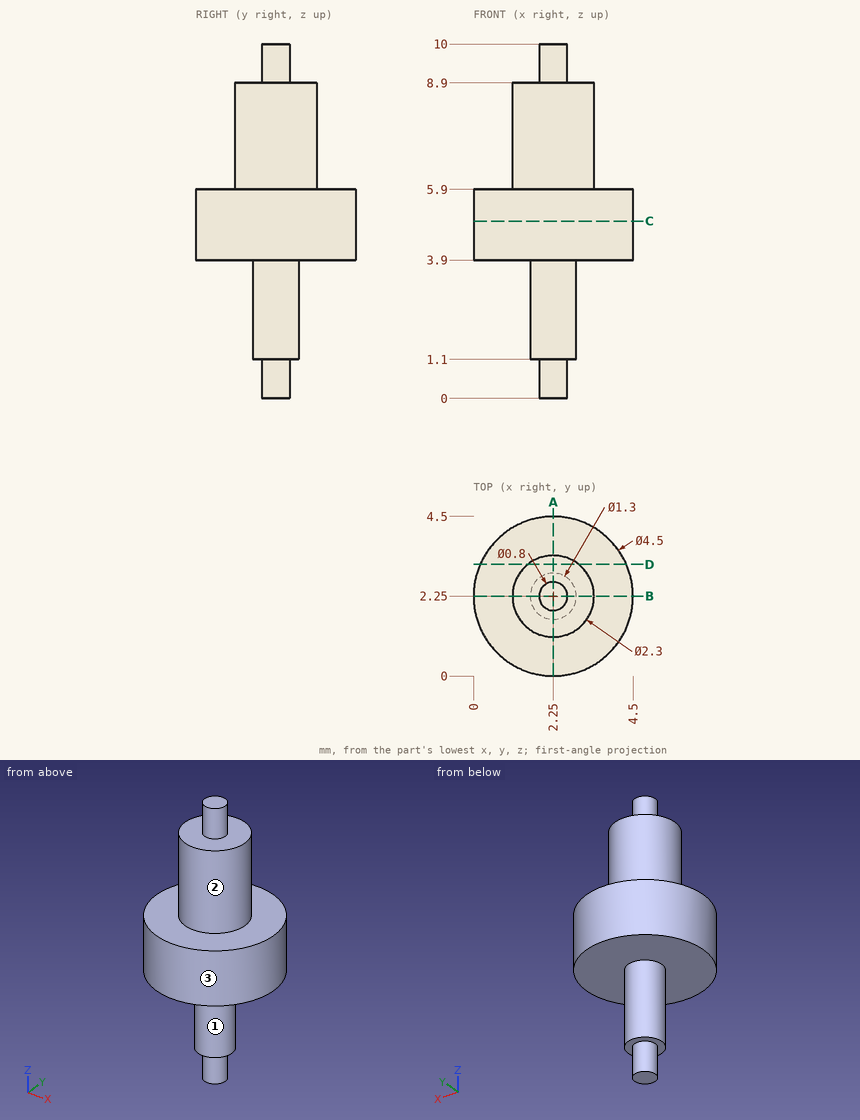
Source: three-view drawing plus pictorial views. Frame: mm from the lowest corner of the part. A direction names the side the tool comes from. Round coordinates to 2 decimals unless told otherwise and drop trailing zeros. Write each loop counter-clockwise with the first axis right and the second up, starting at its lowest first coordinate (ties: lowest second). Pieces come first, ordered by that corner, then holes. Notation, with made-up numbers: M 1.25,56 L 10.25,56 A35 cw 10.25,90 Z; hole C 59.5,7.5 d6. An arc over 180 degrees is marked long. One line per item, written item: value. Start each with the question number.
Item 1: Set-up query: the marked faces 1, 2 and 3. Return all of +Z, -Z, +X, -X, +Y, -Y with unobstructed straight access to the full face (end or side cutting, diameter ignored); none if empty.
Item 2: Section query D-D (y = 3.15). Return the cut outline in (x, z), plus the area to 3 significant figures.
Item 3: Section query A-A (x = 2.25). Return the cut outline in (y, z).
Item 4: Ray query, L1, parallel to Z at x = 4.1, y = 1.45; L2, parallel to Z at x = 1.8, y = 2.6; L3, parallel to Y at x = 1.3, z = 4.5. Return the intervals inside material, ascending. Write a range as from..to.
Item 5: Pin query (flat end, axial travel): pin 1 (2 mm diameter, centred on x = 3, z = 2.5, fed in from -Y); pin 2 (1.5 mm diameter, centred on x = 2.5, z = 8, fed in from -Y); pin 3 (1 mm diameter, centred on x = 1.5, y = 1.5, fed in from -Z); pin 4 (1.4 mm diameter, centred on x = 2, y = 2.5, fed in from -Z). Return the tip coordinate at first contact, or that it passes through.
Item 6: Section query C-C (z = 5). Return the cut outline in (x, y), plus the area to 3 significant figures.
Result set:
1. face 1: -Z
1. face 2: +Z
1. face 3: +Z, -Z
2. outline: M 0.19,3.9 L 4.31,3.9 L 4.31,5.9 L 2.97,5.9 L 2.97,8.9 L 1.53,8.9 L 1.53,5.9 L 0.19,5.9 Z
2. area: 12.5 mm²
3. outline: M 0,3.9 L 1.6,3.9 L 1.6,1.1 L 1.85,1.1 L 1.85,0 L 2.65,0 L 2.65,1.1 L 2.9,1.1 L 2.9,3.9 L 4.5,3.9 L 4.5,5.9 L 3.4,5.9 L 3.4,8.9 L 2.65,8.9 L 2.65,10 L 1.85,10 L 1.85,8.9 L 1.1,8.9 L 1.1,5.9 L 0,5.9 Z
4. L1: z = 3.9..5.9
4. L2: z = 1.1..8.9
4. L3: y = 0.21..4.29
5. pin 1: stops at y = 1.6
5. pin 2: stops at y = 1.1
5. pin 3: stops at z = 1.1
5. pin 4: stops at z = 0
6. outline: C 2.25,2.25 d4.5
6. area: 15.9 mm²
